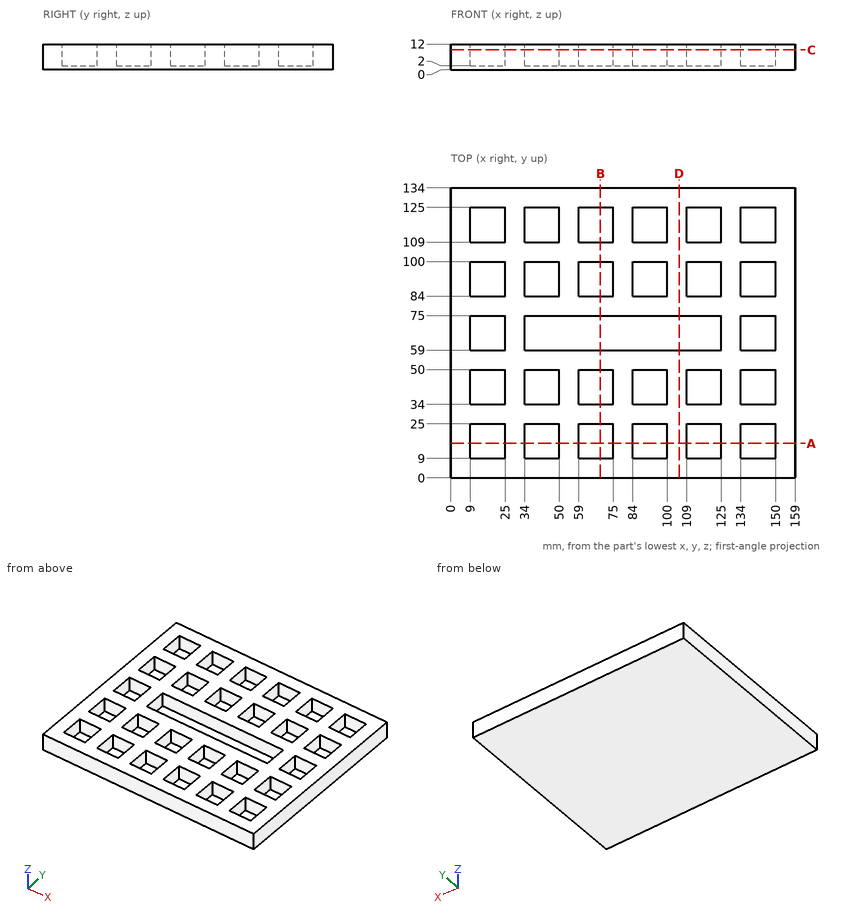
Input: dimensioned drawing with shaded views. Units: mm. Origin: part minimum x, y, z. Give positions to 0.01 mm unless a question says otherwise; leave off trailing zeros. Write each loop counter-clockwise with the first axis right and the second up, starting at its lowest first coordinate (ties: lowest second). Pieces come first, ordered by that corner, then holes.
1. Section query B-B (x = 69). Return the cut outline in (y, z), then the cut area to 3 significant figures.
2. Section query A-A (y = 16). Return the cut outline in (x, z), then the cut area to 3 significant figures.
3. Material intervals for line 1 along Y through (x, z) = (116, 3.75); line 2 along X through (y, z) = (63, 6.5); line 3 along Z through (x, y) = (101.5, 72.5), sorted ascending.
4. Section query C-C (z = 9.25). Count the separate pieces of the cut face and the enclosed holes in it, then the cut area to 3 significant figures.
5. First-contact query: pin 1 (8 mm diameter, centred on x = 94, y = 15.5, fed in from +Z). Flat tip, straight axial feed; report the tip coordinate or a pass-through.
6. Section query D-D (x = 105.5). Return the cut outline in (y, z), then the cut area to 3 significant figures.
Output values:
1. outline: (0, 0) - (134, 0) - (134, 12) - (125, 12) - (125, 2) - (109, 2) - (109, 12) - (100, 12) - (100, 2) - (84, 2) - (84, 12) - (75, 12) - (75, 2) - (59, 2) - (59, 12) - (50, 12) - (50, 2) - (34, 2) - (34, 12) - (25, 12) - (25, 2) - (9, 2) - (9, 12) - (0, 12) - close
1. area: 808 mm2
2. outline: (0, 0) - (159, 0) - (159, 12) - (150, 12) - (150, 2) - (134, 2) - (134, 12) - (125, 12) - (125, 2) - (109, 2) - (109, 12) - (100, 12) - (100, 2) - (84, 2) - (84, 12) - (75, 12) - (75, 2) - (59, 2) - (59, 12) - (50, 12) - (50, 2) - (34, 2) - (34, 12) - (25, 12) - (25, 2) - (9, 2) - (9, 12) - (0, 12) - close
2. area: 948 mm2
3. line 1: y = 0 to 9, 25 to 34, 50 to 59, 75 to 84, 100 to 109, 125 to 134
3. line 2: x = 0 to 9, 25 to 34, 125 to 134, 150 to 159
3. line 3: z = 0 to 2
4. separate pieces: 1
4. enclosed holes: 27
4. area: 13,200 mm2
5. pin 1: stops at z = 2
6. outline: (0, 0) - (134, 0) - (134, 12) - (75, 12) - (75, 2) - (59, 2) - (59, 12) - (0, 12) - close
6. area: 1,450 mm2
